Here's how the part is built. I have some questions about the finished solid (model axes, mm). Give positions to 0.01 mm unless a question says otherwise; leave off trailing zeros. Write each loop counter-clockwise with the first axis right and the second up, starting at its lowest first coordinate (ties: lowest second). Pieces come first, ordered by that corner, then holes. Notation, with made-up numbers: (18, -7) - (25, -7) arc R24 ccw to (25, 17) - close; hole circle Ø11 at (-32.5, 8). An arc over 180 degrees is marked (long way). Use a Markdown table: item, result.
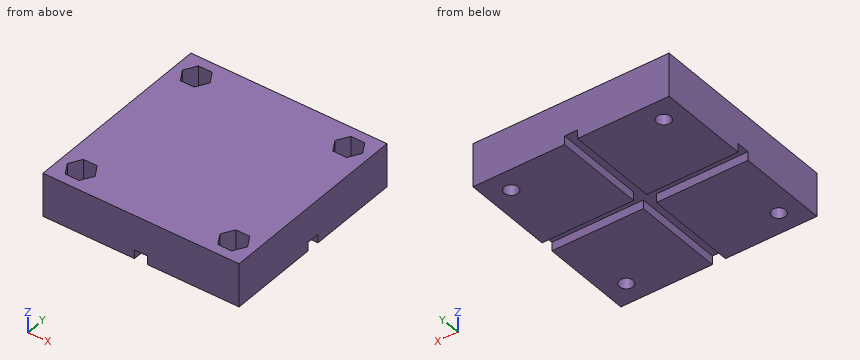
```python
from build123d import *

# Parameters (mm, degrees)
SKETCH1_W           = 45
SKETCH1_H           = 45
SKETCH1_R           = 1.6
BOSS_EXTRUDE1_DEPTH = 10
CUT_EXTRUDE1_DEPTH  = 5
CUT_EXTRUDE2_DEPTH  = 2


with BuildPart() as part:
    # Sketch1 → Boss-Extrude1 (new body)
    with BuildSketch(Plane.XY):
        with Locations((22.5, 22.5)):
            Rectangle(SKETCH1_W, SKETCH1_H)
        with Locations((5, 5)):
            Circle(SKETCH1_R, mode=Mode.SUBTRACT)
        with Locations((5, 40)):
            Circle(SKETCH1_R, mode=Mode.SUBTRACT)
        with Locations((40, 40)):
            Circle(SKETCH1_R, mode=Mode.SUBTRACT)
        with Locations((40, 5)):
            Circle(SKETCH1_R, mode=Mode.SUBTRACT)
    extrude(amount=BOSS_EXTRUDE1_DEPTH)

    # Sketch2 → Cut-Extrude1 (cut)
    with BuildSketch(Plane.XY.offset(10)):
        Polygon((8.175426481, 5), (6.58771324, 7.75), (3.41228676, 7.75), (1.824573519, 5), (3.41228676, 2.25), (6.58771324, 2.25), align=None)
        Polygon((8.175426481, 40), (6.58771324, 42.75), (3.41228676, 42.75), (1.824573519, 40), (3.41228676, 37.25), (6.58771324, 37.25), align=None)
        Polygon((43.175426481, 40), (41.58771324, 42.75), (38.41228676, 42.75), (36.824573519, 40), (38.41228676, 37.25), (41.58771324, 37.25), align=None)
        Polygon((43.175426481, 5), (41.58771324, 7.75), (38.41228676, 7.75), (36.824573519, 5), (38.41228676, 2.25), (41.58771324, 2.25), align=None)
    extrude(amount=-CUT_EXTRUDE1_DEPTH, mode=Mode.SUBTRACT)

    # Sketch3 → Cut-Extrude2 (cut)
    with BuildSketch(Plane(origin=(0, 0, 0), x_dir=(-1, 0, 0), z_dir=(0, 0, -1))):
        Polygon((-45, 24), (-24, 24), (-24, 45), (-21, 45), (-21, 24), (0, 24), (0, 21), (-21, 21), (-21, 0), (-24, 0), (-24, 21), (-45, 21), align=None)
    extrude(amount=-CUT_EXTRUDE2_DEPTH, mode=Mode.SUBTRACT)


solid = part.part
```
Item 1: Will these pins go through, and if not, where does the flat tip stop? pin 1 Ø1.6 at (x, y) = (5.5, 4) entering from +Z; pin 2 Ø12 at (x, y) = (19, 22.5) entering from -Z.
Values:
| item | result |
|---|---|
| pin 1 | stops at z = 5 |
| pin 2 | stops at z = 0 |
Item 2: If we section it at A-A, the plane x = 5: Write out the boundary of the cut face in (y, z).
Values:
| item | result |
|---|---|
| outline | (0, 0) - (3.4, 0) - (3.4, 5) - (2.25, 5) - (2.25, 10) - (0, 10) - close; (6.6, 0) - (21, 0) - (21, 2) - (24, 2) - (24, 0) - (38.4, 0) - (38.4, 5) - (37.25, 5) - (37.25, 10) - (7.75, 10) - (7.75, 5) - (6.6, 5) - close; (41.6, 0) - (45, 0) - (45, 10) - (42.75, 10) - (42.75, 5) - (41.6, 5) - close |
Item 3: I need wall thicknesses on line 1 along X through (y, z) = (5, 3.85); line 2 along Y through (x, z) = (39, 5.75). Which ranges of each line are inside material? Lowest first, please. Write a range as [from, to].
Values:
| item | result |
|---|---|
| line 1 | x = [0, 3.4], [6.6, 38.4], [41.6, 45] |
| line 2 | y = [0, 2.25], [7.75, 37.25], [42.75, 45] |
Item 4: If we section it at B-B, the plane z = 6.5: Write out the boundary of the cut face in (x, y), plus the area to 3 significant figures.
Values:
| item | result |
|---|---|
| outline | (0, 0) - (45, 0) - (45, 45) - (0, 45) - close; hole (1.82, 5) - (3.41, 2.25) - (6.59, 2.25) - (8.18, 5) - (6.59, 7.75) - (3.41, 7.75) - close; hole (1.82, 40) - (3.41, 37.25) - (6.59, 37.25) - (8.18, 40) - (6.59, 42.75) - (3.41, 42.75) - close; hole (36.82, 5) - (38.41, 2.25) - (41.59, 2.25) - (43.18, 5) - (41.59, 7.75) - (38.41, 7.75) - close; hole (36.82, 40) - (38.41, 37.25) - (41.59, 37.25) - (43.18, 40) - (41.59, 42.75) - (38.41, 42.75) - close |
| area | 1,920 mm2 |
